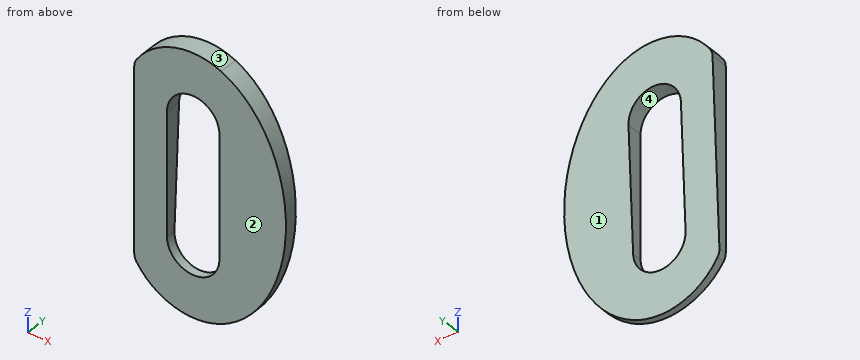
Autodesk Inventor part; units mm, degrees
ref_plane "YZ Plane" through (0, 0, 0) normal (1, 0, 0) x (0, 1, 0)
ref_plane "XZ Plane" through (0, 0, 0) normal (0, 1, 0) x (-1, 0, 0)
ref_plane "XY Plane" through (0, 0, 0) normal (0, 0, 1) x (1, 0, 0)
sketch "Sketch1" plane through (0, 0, 0) normal (0, 1, 0) x (-1, 0, 0)
  line L0 (0, 0) -> (0, -34.15) construction
  arc A0 (6.6649, -3.975) -> (-7.575, -7.575) centre (0, -7.575) ccw construction
  arc A1 (-7.575, -26.575) -> (6.6649, -30.175) centre (0, -26.575) ccw construction
  line L1 (4.075, -7.575) -> (4.075, -26.575) construction
  arc A2 (-4.075, -26.575) -> (4.075, -26.575) centre (0, -26.575) ccw construction
  line L2 (-4.075, -26.575) -> (-4.075, -7.575) construction
  arc A3 (4.075, -7.575) -> (-4.075, -7.575) centre (0, -7.575) ccw construction
  line L3 (9.1649, -3.975) -> (9.1649, -30.175) construction
  line L4 (9.1649, -3.975) -> (6.6649, -3.975) construction
  line L5 (9.1649, -30.175) -> (6.6649, -30.175) construction
  line L6 (-10.575, -14.075) -> (-10.575, -20.075) construction
  line L7 (0, -17.075) -> (-19.3792, -17.075) construction
  line L8 (-4.075, -20.075) -> (-4.075, -24.075) construction
  line L9 (-10.575, -20.075) -> (-7.575, -21.8932) construction
  line L10 (-10.575, -14.075) -> (-7.575, -12.2568) construction
  line L11 (-7.575, -7.575) -> (-7.575, -12.2568) construction
  line L12 (-7.575, -21.8932) -> (-7.575, -26.575) construction
  line L13 (-10.575, -17.075) -> (-16.875, -17.075) construction
  line L14 (-10.575, -14.075) -> (-14.875, -14.075) construction
  line L15 (-16.875, -16.075) -> (-16.875, -18.075) construction
  line L16 (-14.875, -20.075) -> (-10.575, -20.075) construction
  arc A4 (-14.875, -14.075) -> (-16.875, -16.075) centre (-14.875, -16.075) ccw construction
  arc A5 (-16.875, -18.075) -> (-14.875, -20.075) centre (-14.875, -18.075) ccw construction
  line L17 (-6.7059, -17.075) -> (-6.7059, -23.075) construction
  line L18 (-6.7059, -17.075) -> (-6.7059, -11.075) construction
  line L19 (-7.575, -11.075) -> (-14.875, -11.075) construction
  line L20 (-16.875, -13.075) -> (-16.875, -21.075) construction
  line L21 (-14.875, -23.075) -> (-7.575, -23.075) construction
  arc A6 (-14.875, -11.075) -> (-16.875, -13.075) centre (-14.875, -13.075) ccw construction
  arc A7 (-16.875, -21.075) -> (-14.875, -23.075) centre (-14.875, -21.075) ccw construction
  line L22 (19.3047, -16.075) -> (19.3047, -18.075) construction
  line L23 (17.3047, -14.075) -> (13.3047, -14.075) construction
  line L24 (17.3047, -20.075) -> (13.3047, -20.075) construction
  line L25 (9.1649, -16.075) -> (9.1649, -22.575) construction
  line L26 (9.1649, -17.075) -> (9.1649, -11.575) construction
  line L27 (9.1649, -11.575) -> (13.3047, -14.075) construction
  line L28 (9.1649, -22.575) -> (13.3047, -20.075) construction
  arc A8 (19.3047, -16.075) -> (17.3047, -14.075) centre (17.3047, -16.075) ccw construction
  arc A9 (17.3047, -20.075) -> (19.3047, -18.075) centre (17.3047, -18.075) ccw construction
  line L29 (9.1649, -30.175) -> (9.1649, -26.175) construction
  line L30 (9.1649, -3.975) -> (9.1649, -7.975) construction
  line L31 (9.1649, -24.9114) -> (13.8618, -22.075) construction
  line L32 (13.8618, -22.075) -> (17.3047, -22.075) construction
  arc A10 (17.3047, -22.075) -> (21.3047, -18.075) centre (17.3047, -18.075) ccw construction
  line L33 (21.3047, -18.075) -> (21.3047, -16.075) construction
  arc A11 (21.3047, -16.075) -> (17.3047, -12.075) centre (17.3047, -16.075) ccw construction
  line L34 (17.3047, -12.075) -> (13.8618, -12.075) construction
  line L35 (13.8618, -12.075) -> (9.1649, -9.2386) construction
  point P0 (7.575, -17.075)
  point P1 (-4.075, -10.075)
  point P2 (19.3047, -14.075)
  point P3 (19.3047, -20.075)
  dimension "d0" = 34.15
  dimension "d1" = 15.15
  dimension "d5" = 6
  dimension "d7" = 4
  dimension "d8" = 2.5
  dimension "d9" = 3.5
  dimension "d10" = 8.15
  dimension "d12" = 2
  dimension "d14" = 6
  dimension "d15" = 6
  dimension "d16" = 2
  dimension "d18" = 6
  dimension "d19" = 6
  dimension "d20" = 5.5
  dimension "d21" = 5.5
  dimension "d23" = 4
  dimension "d24" = 4
  dimension "d25" = 2
sketch "Sketch3" plane through (0, 0, 0) normal (0, 1, 0) x (-1, 0, 0)
  arc A0 (6.6649, -3.975) -> (-7.575, -7.575) centre (0, -7.575) ccw construction
  arc A1 (-7.575, -26.575) -> (6.6649, -30.175) centre (0, -26.575) ccw construction
  arc A2 (-4.075, -26.575) -> (4.075, -26.575) centre (0, -26.575) ccw
  line L0 (4.075, -7.575) -> (4.075, -26.575)
  arc A3 (4.075, -7.575) -> (-4.075, -7.575) centre (0, -7.575) ccw
  line L1 (-4.075, -26.575) -> (-4.075, -7.575)
  line L2 (9.1649, -3.975) -> (9.1649, -30.175) construction
  line L3 (-10.575, -14.075) -> (-10.575, -20.075) construction
  line L4 (-16.875, -16.075) -> (-16.875, -18.075) construction
  arc A4 (8.836, -1.765) -> (-4.3309, 2.0725) centre (0, -7.575) ccw
  arc A5 (-4.3309, -36.2225) -> (8.836, -32.385) centre (0, -26.575) ccw
  line L5 (9.1649, -2.8638) -> (9.1649, -31.2862)
  arc A6 (9.1649, -2.8638) -> (8.836, -1.765) centre (7.1649, -2.8638) ccw
  arc A7 (8.836, -32.385) -> (9.1649, -31.2862) centre (7.1649, -31.2862) ccw
  line L6 (-12.075, -10.8843) -> (-12.075, -24.6972)
  ellipse E0 centre (0, -17.075) end of major axis (0, -37.15) minor radius 14.4147 (-4.3309, 2.0725) -> (-4.3309, -36.2225) ccw
  point P0 (0, 0)
  point P1 (9.1649, -2.2991)
  point P2 (9.1649, -31.8509)
  dimension "d26" = 3
  dimension "d27" = 3
  dimension "d28" = 2
  dimension "d29" = 6.5
  dimension "d30" = 8
extrude "Extrusion1" add sketch "Sketch3" along normal blind 3
ref_plane "Work Plane1" through (0, 1, 3) normal (1, 0, 0) x (0, 0, -1)
sketch "Sketch8" plane through (0, 1, 3) normal (1, 0, 0) x (0, 0, -1)
  line L0 (40.15, 2) -> (40.15, -1)
  line L1 (40.15, -1) -> (33.65, -1)
  line L2 (33.65, -1) -> (33.65, 2)
  line L3 (33.65, 2) -> (40.15, 2)
  line L4 (0, -1) -> (0, 2)
  line L5 (0, 2) -> (6.5, 2)
  line L6 (6.5, 2) -> (6.5, -1)
  line L7 (6.5, -1) -> (0, -1)
  line L8 (40.15, -1) -> (40.15, 0)
  line L9 (40.15, -1) -> (40.15, 2)
  line L10 (40.15, 0) -> (0, 2)
  line L11 (4.765, 2) -> (0, 2)
  line L12 (40.15, 2) -> (35.385, 2)
  line L13 (0, 2) -> (40.15, 2)
  line L14 (40.15, 2) -> (40.15, 0)
  point P0 (3, -1)
  point P1 (0.9275, 2)
  point P2 (39.2225, 2)
  dimension "d38" = 1
extrude "Extrusion3" cut sketch "Sketch8" along normal blind 30 and the other way blind 30 contours L0 L10 L2 L3 | L10 L6 L13 L2 | L10 L5 L6
properties part number "SPD_MTB_cleat_new_3mm_01mm"
Part model, mm, in its own coordinate system. Face numbers are marked on the shaded views. Round coordinates to 2 decimals unless told otherwise and drop trailing zeros. Write each loop counter-clockwise with the first axis right and the second up, starting at its lowest first coordinate (ties: lowest second). Pieces come first, ordered by that corner, then holes. Notation, with made-up numbers: M 14.5,-31.75 L 51.5,-31.75 A12 ccw 51.5,-11.75 Z; hole C 78.5,67.25 d6. An arc over 180 degrees is marked long. Answer as CSV lines item,"result". Start each with the question number.
1) Drop flat-ended pins along their axis: pin 1 (1 mm diameter, centred on x = 9.5, z = -13.5, fed in from +Y); pin 2 (12 mm diameter, centred on x = 11, z = -26.5, fed in from +Y); pin 3 (1 mm diameter, centred on x = 11, y = 1.5, fed in from +Z). Give the stop position or say it passes through.
2) Drill centre lines: L1, parallel to Z at x = 0, y = 0.65; L2, parallel to Z at x = 1.5, y = 0.5; L3, parallel to X at y = 0.7, z = -10 (3 decimals). Where is each one in solid material? Low to high.
3) Band-saw the part on A-A (x = 1.25). List the corners of the cut face in (y, z), then the cut area to 3 significant figures.
4) Mould opens along Z. For the marked faces 1, 2, 3 and 4 say: +Z half, -Z half, draft (parallel to the pull), parting line (faces both ways), or undercut.
5) Band-saw the part on B-B (x = -3.5). List the corners of the cut face in (y, z), then the cut area to 3 significant figures.
6) Band-saw the part on C-C (x = -6.75). List the corners of the cut face in (y, z), then the cut area to 3 significant figures.
Worked out:
1,pin 1,"y = 2.2"
1,pin 2,"y = 1.83"
1,pin 3,"z = -3.32"
2,L1,"-37.15 to -30.65, -3.5 to 3"
2,L2,"-37.04 to -30.36, -3.79 to 2.89"
2,L3,"-9.165 to -4.075, 4.075 to 13.49"
3,outline,"M 0,-37.08 L 1,-37.08 L 1.33,-30.45 L 0,-30.45 Z; M 0,-3.7 L 2.67,-3.7 L 3,2.93 L 0,2.93 Z"
3,area,"26.5 mm²"
4,face 1,"-Z half"
4,face 2,"draft"
4,face 3,"+Z half"
4,face 4,"undercut"
5,outline,"M 0,-36.55 L 1.03,-36.55 L 1.42,-28.66 L 0,-28.66 Z; M 0,-5.49 L 2.58,-5.49 L 2.97,2.4 L 0,2.4 Z"
5,area,"31.6 mm²"
6,outline,"M 0,-34.72 L 1.12,-34.72 L 2.88,0.57 L 0,0.57 Z"
6,area,"70.6 mm²"
